Source: CAD feature listing. Evaluate the final solid. Frame: model axes, mm. Face numbers are marked on the shaded views. A direction names the side the tool comes from. Round coordinates to 2 decimals unless told otherwise and drop trailing zeros. Loops run counter-clockwise (first coordinate to the right, second up) from the corner with the lowest first, then second, coordinate; pieces in that order, holes last.
Item 1: Section query B-B on x = 61.5. Return loops of the section in (y, z), then the cut area to 3 significant figures.
Item 2: Section query C-C on x = 26. Return loops of the section in (y, z).
Item 3: First-contact query: P1, Ø12, axis at y = -16, z = 24, coming from the +X side; P2, Ø10, axis at x = 37, z = 31.5, coming from the +Y side; P3, Ø5, axis at y = -15.5, z = 23, coming from the +X side; P4, Ø3.5, axis at x = 69.5, y = -15, coming from the +Z side. Flat tips, straight axial feed; report the tip coordinate or a pass-through.
Item 4: Ray query, L1, parallel to X at y = -1.5, z = 43; L2, parallel to Y at x = 72.5, z = 44; L3, parallel to Z at x = 50.5, y = -5.25. Return the intervals inside material, ascending.
Item 5: Access query for the marked faces 4, 5 and 6. Directions: +Z, -Z, +X, -X, +Y, -Y. A direction counts if a zero-diameter tool reaches every point of the face in a straight line with its end or side. Return the directions, or none.
Item 6: Section query A-A on z = 42. Return loops of the section in (x, y).
Item 7: Pull-direction query (Y, two-part tool) for the marked faces 1, 2 and 3; classes: released by +Y, released by -Y, zero draft, split by the parting line, or undercut.
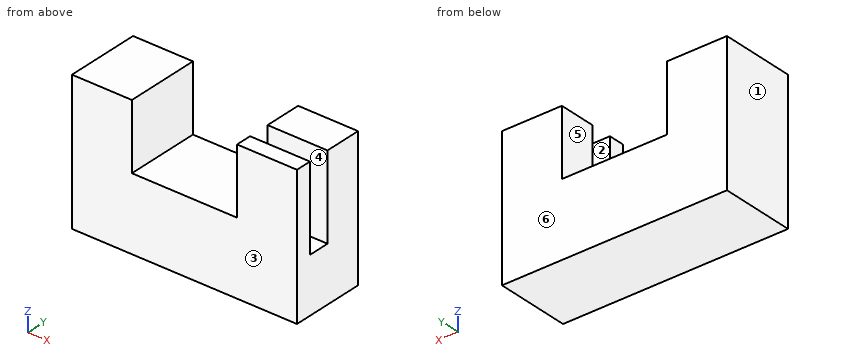
```python
from build123d import *

# Parameters (mm, degrees)
F1_DEPTH = 25.4
F2_W     = 20.367536
F2_H     = 9.66201
F3_DEPTH = 25.4
F4_W     = 8.65579
F4_H     = 21.259759
F5_DEPTH = 25.146
F6_W     = 20.367536
F6_H     = 7.306238
F7_DEPTH = 28.702


with BuildPart() as f1:
    # F0 (on Front) → F1 (new body)
    with BuildSketch(Plane.XZ):
        Polygon((20.367537, 47.451993), (0, 47.451993), (0, 0), (76.48655, 0), (76.48655, 47.451993), (56.119014, 47.451993), (56.119014, 24.917716), (20.367537, 24.917716), align=None)
    extrude(amount=F1_DEPTH)

    # F2 (on face) → F3 (cut)
    with BuildSketch(Plane.XY.offset(47.451993)):
        with Locations((66.302782, -14.511633)):
            Rectangle(F2_W, F2_H)
    extrude(amount=F3_DEPTH, mode=Mode.SUBTRACT)

    # F4 (on face) → F5 (join)
    with BuildSketch(Plane.XY.offset(47.451993)):
        with Locations((66.302782, -14.77012)):
            Rectangle(F4_W, F4_H)
    extrude(amount=-F5_DEPTH)

    # F6 (on face) → F7 (cut)
    with BuildSketch(Plane.XY.offset(47.451993)):
        with Locations((66.302782, -16.353119)):
            Rectangle(F6_W, F6_H)
    extrude(amount=-F7_DEPTH, mode=Mode.SUBTRACT)


solid = f1.part
```
Data:
1. outline: (-25.4, 0) - (0, 0) - (0, 47.45) - (-12.7, 47.45) - (-12.7, 18.75) - (-20.01, 18.75) - (-20.01, 47.45) - (-25.4, 47.45) - close
1. area: 996 mm2
2. outline: (-25.4, 0) - (0, 0) - (0, 24.92) - (-25.4, 24.92) - close
3. P1: stops at x = 76.49
3. P2: passes through
3. P3: stops at x = 56.12
3. P4: stops at z = 18.75
4. L1: x = 0 to 20.37, 56.12 to 76.49
4. L2: y = -25.4 to -20.01, -12.7 to 0
4. L3: z = 0 to 24.92
5. face 4: +Z, +X
5. face 5: +Z, +Y, -Y
5. face 6: +Z, -Z, +X, -X, +Y
6. outline: (0, -25.4) - (20.37, -25.4) - (20.37, 0) - (0, 0) - close; (56.12, -25.4) - (76.49, -25.4) - (76.49, -20.01) - (56.12, -20.01) - close; (56.12, -12.7) - (76.49, -12.7) - (76.49, 0) - (56.12, 0) - close
7. face 1: zero draft
7. face 2: undercut
7. face 3: released by -Y
